For this review, take the finished solid that the model builds, in its own axes (mm). Face numbers are marked on the shaded views. Coordinates: 2 decimals unless noted, no trailing zeros. Loops run counter-clockwise (first coordinate to the right, second up) from the corner with the lowest first, then second, coordinate; pieces in that order, holes last. Notation, with made-up numbers: (-33, 44.5) - (20, 44.5) arc R18 ccw to (20, 63.5) - close; hole circle Ø5 at (-23.5, 67). An arc over 180 degrees is marked (long way). Answer as a JSON object with one key per item and string values. Group by question number.
Item 1: To check wall thickness, follow line 1 (X direction, y = 8, z = -19); line 2 (Y direction, x = 56, z = 1); line 3 (Z direction, x = 27, y = 23.5). State the ranges of each line that lie inside material, in increasing order.
Item 2: Clearance check with flat-ended pins moving along their axes: pin 1 (10 mm diameter, centred on x = 112.5, y = 16, fed in from -Z); pin 2 (6 mm diameter, centred on x = 30, z = -47.5, fed in from +Y); pin 3 (1 mm diameter, centred on y = 5, z = -26.5, fed in from +X). State where each tip first meets the part, or that it passes through.
Item 3: We need section B-B (x = 38). Give the boundary of the cut face in (y, z), then the cut area to 3 significant figures.
Item 4: We need section A-A (y = 31.5). State how many separate pieces and enclosed holes the cut face has, then the cut area to 3 significant figures.
Item 5: Mouldability with a two-part tool opening along Z and no side actions: class the marked faces 1, 2 and 3 as released by +Z, released by -Z, zero draft, split by the parting line, or undercut.
Item 6: We need section D-D (z = -91). Give the boundary of the cut face in (x, y).
from build123d import *

# Parameters (mm, degrees)
SKETCH1_W           = 127.635
SKETCH1_H           = 127.635
MAIN_PLATE_DEPTH    = 12.7
SKETCH9_R           = 85.725
BOSS_EXTRUDE1_DEPTH = 12.7
SKETCH10_R          = 95.25
SKETCH10_R_2        = 85.4075
CUT_EXTRUDE1_DEPTH  = 167.64
SKETCH18_R          = 85.4075
SKETCH18_R_2        = 79.375
BOSS_EXTRUDE2_DEPTH = 38.1
SKETCH15_R          = 2.159
CUT_EXTRUDE3_DEPTH  = 88.9
CIRPATTERN1_COUNT   = 3
SKETCH21_R          = 15.875
SKETCH21_R_2        = 1.778
CO2_MOUNTS_DEPTH    = 13.7000001
SKETCH22_R          = 5.08
CUT_EXTRUDE5_DEPTH  = 13.7000001
SKETCH23_R          = 79.375
CUT_EXTRUDE6_DEPTH  = 111.600000066


with BuildPart() as part:
    # Sketch1 → Main Plate (new body)
    with BuildSketch(Plane(origin=(0, 0, 0), x_dir=(1, 0, 0), z_dir=(0, 1, 0))):
        with Locations((63.8175, 63.8175)):
            Rectangle(SKETCH1_W, SKETCH1_H)
    extrude(amount=MAIN_PLATE_DEPTH)

    # Sketch9 → Boss-Extrude1 (add)
    with BuildSketch(Plane(origin=(0, 12.7, 0), x_dir=(1, 0, 0), z_dir=(0, 1, 0))):
        with Locations((63.8175, 63.8175)):
            Circle(SKETCH9_R)
    extrude(amount=-BOSS_EXTRUDE1_DEPTH)

    # Sketch10 → Cut-Extrude1 (cut)
    with BuildSketch(Plane(origin=(0, 12.7, 0), x_dir=(1, 0, 0), z_dir=(0, 1, 0))):
        with Locations((63.8175, 63.8175)):
            Circle(SKETCH10_R)
        with Locations((63.8175, 63.8175)):
            Circle(SKETCH10_R_2, mode=Mode.SUBTRACT)
    extrude(amount=-CUT_EXTRUDE1_DEPTH, mode=Mode.SUBTRACT)

    # Sketch18 → Boss-Extrude2 (add)
    with BuildSketch(Plane(origin=(0, 6.35, 0), x_dir=(1, 0, 0), z_dir=(0, 1, 0))):
        with Locations((63.8175, 63.8175)):
            Circle(SKETCH18_R)
        with Locations((63.8175, 63.8175)):
            Circle(SKETCH18_R_2, mode=Mode.SUBTRACT)
    extrude(amount=BOSS_EXTRUDE2_DEPTH)

    # Sketch15 → Cut-Extrude3 (cut)
    with BuildSketch(Plane(origin=(166.221610148, 0, 178.614251028), x_dir=(-0.866025404, 0, -0.5), z_dir=(0.5, 0, -0.866025404))):
        with Locations((209.900436354, 22.225)):
            Circle(SKETCH15_R)
        with Locations((209.900436354, 38.1)):
            Circle(SKETCH15_R)
        with Locations((209.900436354, 6.35)):
            Circle(SKETCH15_R)
    cut_extrude3 = extrude(amount=CUT_EXTRUDE3_DEPTH, mode=Mode.SUBTRACT)

    # CirPattern1: Cut-Extrude3 ×3 about axis
    cirpattern1_axis = Axis((63.8175, 0, -63.8175), (0, 1, 0))
    for i in range(1, CIRPATTERN1_COUNT):
        add(cut_extrude3.rotate(cirpattern1_axis, i * 360 / CIRPATTERN1_COUNT), mode=Mode.SUBTRACT)

    # Sketch21 → CO2 Mounts (cut, through all)
    with BuildSketch(Plane(origin=(0, 12.7, 0), x_dir=(1, 0, 0), z_dir=(0, 1, 0))):
        with Locations((102.235, 63.8175)):
            Circle(SKETCH21_R)
        with Locations((102.235, 82.8675)):
            Circle(SKETCH21_R_2)
        with Locations((25.4, 63.8175)):
            Circle(SKETCH21_R)
        with Locations((121.285, 63.8175)):
            Circle(SKETCH21_R_2)
        with Locations((102.235, 44.7675)):
            Circle(SKETCH21_R_2)
        with Locations((83.185, 63.8175)):
            Circle(SKETCH21_R_2)
        with Locations((25.4, 82.8675)):
            Circle(SKETCH21_R_2)
        with Locations((6.35, 63.8175)):
            Circle(SKETCH21_R_2)
        with Locations((25.4, 44.7675)):
            Circle(SKETCH21_R_2)
        with Locations((44.45, 63.8175)):
            Circle(SKETCH21_R_2)
    extrude(amount=-CO2_MOUNTS_DEPTH, mode=Mode.SUBTRACT)

    # Sketch22 → Cut-Extrude5 (cut, through all)
    with BuildSketch(Plane(origin=(0, 12.7, 0), x_dir=(1, 0, 0), z_dir=(0, 1, 0))):
        with Locations((46.355, 108.585)):
            Circle(SKETCH22_R)
        with Locations((81.28, 108.585)):
            Circle(SKETCH22_R)
        with Locations((81.28, 19.05)):
            Circle(SKETCH22_R)
        with Locations((46.355, 19.05)):
            Circle(SKETCH22_R)
    extrude(amount=-CUT_EXTRUDE5_DEPTH, mode=Mode.SUBTRACT)

    # Sketch23 → Cut-Extrude6 (cut)
    with BuildSketch(Plane(origin=(0, 12.7, 0), x_dir=(1, 0, 0), z_dir=(0, 1, 0))):
        with Locations((63.8175, 63.8175)):
            Circle(SKETCH23_R)
        with BuildLine():
            Line((13.678739997, 125.352005526), (7.552270878, 134.237860218))
            Line((7.552270878, 134.237860218), (-19.267108419, 125.320629884))
            Line((-19.267108419, 125.320629884), (-48.79695837, 60.397770071))
            Line((-48.79695837, 60.397770071), (-9.884344094, 7.052469015))
            Line((-9.884344094, 7.052469015), (6.959175986, -7.46308736))
            Line((6.959175986, -7.46308736), (13.678739997, 2.282994474))
            ThreePointArc((13.678739997, 2.282994474), (-15.5575, 63.8175), (13.678739997, 125.352005526))
        make_face()
        with BuildLine():
            Line((142.177324996, 76.471687114), (152.935935453, 77.334437661))
            Line((152.935935453, 77.334437661), (158.623077101, 105.019316613))
            Line((158.623077101, 105.019316613), (117.163156193, 163.054346747))
            Line((117.163156193, 163.054346747), (51.508463168, 156.027684783))
            Line((51.508463168, 156.027684783), (30.515862556, 148.698546693))
            Line((30.515862556, 148.698546693), (35.596435007, 138.00619264))
            ThreePointArc((35.596435007, 138.00619264), (103.505, 132.558266425), (142.177324996, 76.471687114))
        make_face()
        with BuildLine():
            Line((35.596435007, -10.37119264), (30.964293669, -20.119797879))
            Line((30.964293669, -20.119797879), (52.096531318, -38.887446496))
            Line((52.096531318, -38.887446496), (123.086302178, -31.999616818))
            Line((123.086302178, -31.999616818), (149.828380926, 28.372346201))
            Line((149.828380926, 28.372346201), (153.977461458, 50.217040667))
            Line((153.977461458, 50.217040667), (142.177324996, 51.163312886))
            ThreePointArc((142.177324996, 51.163312886), (103.505, -4.923266425), (35.596435007, -10.37119264))
        make_face()
    extrude(amount=CUT_EXTRUDE6_DEPTH, mode=Mode.SUBTRACT)


solid = part.part
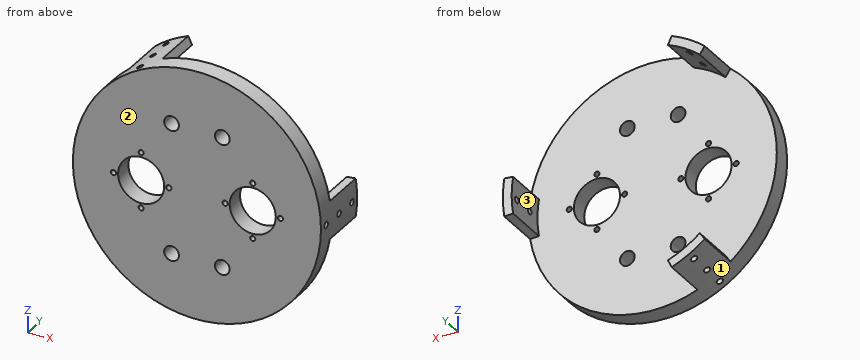
Check sheet entries:
{
 "1": {"line 1": "x = -8.89 to 41.28, 51.43 to 76.2, 86.36 to 136.52", "line 2": "y = 0 to 12.7", "line 3": "z = -140.88 to -134.14, 6.5 to 13.25"},
 "2": {"pin 1": "stops at z = -136.45", "pin 2": "stops at y = 12.7", "pin 3": "stops at x = 140.88"},
 "3": {"outline": "(0, -145.23) - (12.7, -145.23) - (12.7, -73.47) - (0, -73.47) - close; (0, -54.16) - (12.7, -54.16) - (12.7, 17.59) - (0, 17.59) - close", "area": "1,820 mm2"},
 "4": {"separate pieces": "3", "enclosed holes": "0", "area": "469 mm2"},
 "5": {"face 1": "split by the parting line", "face 2": "zero draft", "face 3": "undercut"},
 "6": {"outline": "(-17.15, 0) - (144.78, 0) - (144.78, 12.7) - (-17.15, 12.7) - close"}
}
